from build123d import *

# Parameters (mm, degrees)
BOSS_EXTRUDE1_DEPTH = 24
CUT_EXTRUDE1_DEPTH  = 43
SKETCH7_R           = 12.7
CUT_EXTRUDE4_DEPTH  = 10


with BuildPart() as part:
    # Sketch1 → Boss-Extrude1 (new, symmetric)
    with BuildSketch(Plane.XY):
        with BuildLine():
            Line((0, 41.872855029), (0, -41.872855029))
            ThreePointArc((0, -41.872855029), (5.455474373, -55.600810969), (18.845677428, -61.839515726))
            Line((18.845677428, -61.839515726), (160, -70))
            ThreePointArc((160, -70), (230, 0), (160, 70))
            Line((160, 70), (18.845677428, 61.839515726))
            ThreePointArc((18.845677428, 61.839515726), (5.455474373, 55.600810969), (0, 41.872855029))
        make_face()
    extrude(amount=BOSS_EXTRUDE1_DEPTH, both=True)

    # Sketch2 → Cut-Extrude1 (cut)
    with BuildSketch(Plane(origin=(0, 0, -24), x_dir=(-1, 0, 0), z_dir=(0, 0, -1))):
        with BuildLine():
            Line((-19.134258071, 56.847850552), (-160.141737643, 64.999845465))
            ThreePointArc((-160.141737643, 64.999845465), (-225, 0), (-160.141737643, -64.999845465))
            Line((-160.141737643, -64.999845465), (-19.134258071, -56.847850552))
            ThreePointArc((-19.134258071, -56.847850552), (-9.09160578, -52.168821984), (-5, -41.872855029))
            Line((-5, -41.872855029), (-5, 41.872855029))
            ThreePointArc((-5, 41.872855029), (-9.09160578, 52.168821984), (-19.134258071, 56.847850552))
        make_face()
    extrude(amount=-CUT_EXTRUDE1_DEPTH, mode=Mode.SUBTRACT)

    # Sketch7 → Cut-Extrude4 (cut)
    with BuildSketch(Plane.XY.offset(24)):
        with Locations((50, 0)):
            Circle(SKETCH7_R)
    extrude(amount=-CUT_EXTRUDE4_DEPTH, mode=Mode.SUBTRACT)


solid = part.part
The listing builds one solid part. Answer for the finished solid, in the listing's coordinates (mm). A direction names the side the tool comes from. Coordinates: 2 decimals unless noted, no trailing zeros. Write each loop counter-clockwise with the first axis right and the second up, starting at its lowest first coordinate (ties: lowest second). Pieces come first, ordered by that corner, then holes. Notation, with made-up numbers: M 71.25,22 L 125.25,22 A20 cw 125.25,42 Z; hole C 77.25,25.5 d7. An arc over 180 degrees is marked long. Write each question's results on one line, items separated by ' | '.
Item 1: The part is cut by section B-B on x = 50. Determine the outline of the cut face in (y, z).
Answer below:
outline: M -63.64,-24 L -58.63,-24 L -58.63,19 L -12.7,19 L -12.7,24 L -63.64,24 Z; M 12.7,19 L 58.63,19 L 58.63,-24 L 63.64,-24 L 63.64,24 L 12.7,24 Z
Item 2: The part is cut by section C-C on z = -2.5. Determine the outline of the cut face in (x, y), and give its area (3 significant figures).
Answer below:
outline: M 0,-41.87 A20 ccw 18.85,-61.84 L 160,-70 A70 ccw 160,70 L 18.85,61.84 A20 ccw 0,41.87 Z; hole M 5,-41.87 A15 ccw 19.13,-56.85 L 160.14,-65 A65 ccw 160.14,65 L 19.13,56.85 A15 ccw 5,41.87 Z | area: 3,160 mm2
Item 3: The part is cut by section D-D on y = -46. Determine the outline of the cut face in (x, z), and give its area (3 significant figures).
Answer below:
outline: M 0.43,-24 L 5.58,-24 L 5.58,19 L 205.92,19 L 205.92,-24 L 212.76,-24 L 212.76,24 L 0.43,24 Z | area: 1,580 mm2
Item 4: Which of the six approach directions +Z, -Z, +X, -X, +Y, -Y give full straight-line access (tool end or side, diameter ignored) to faces 1 (the face through (9.2, -52.28, -2.8)), 2 (the face through (88.435, -65.863, 0.336))?
Answer below:
face 1: -Z | face 2: +Z, -Z, -X, -Y
Item 5: For a pull along X with two mould halves and no side action, classify faces 3 (the face through (62.114, 3.815, 21.535)), 4 (the face through (90.411, 65.977, 0.336)), 5 (the face through (113, 1, 24)) as released by +X, released by -X, zero draft, split by the parting line, or undercut.
Answer below:
face 3: undercut | face 4: released by -X | face 5: zero draft
Item 6: Consider probe 1 along Z at (x, y) = (44, 23); probe 2 along X at (y, z) = (13, 16.5); probe 3 along Y at (x, z) = (101, -15.5). Determine where each line is inside the solid, lowest interval first. Write a range as [from, to].
Answer below:
probe 1: [19, 24] | probe 2: [0, 5], [223.69, 228.78] | probe 3: [-66.59, -61.58], [61.58, 66.59]
Item 7: Given P1, Ø8, axis at x = 203, z = -15, coming from the +Y side; P2, Ø2, axis at x = 204.5, z = 7, coming from the -Y side; P3, Ø13, axis at y = -4, z = 3, coming from the +X side; P4, Ø20.5, axis at x = 50, y = 0, coming from the +Z side, each flat-ended and moving along its own axis, determine where each tip first touches the part or whether it passes through.
Answer below:
P1: y = 58.13 | P2: y = -54.84 | P3: x = 230 | P4: through
Item 8: The part is cut by section A-A on y = 0. Determine the outline of the cut face in (x, z), and give its area (3 significant figures).
Answer below:
outline: M 0,-24 L 5,-24 L 5,19 L 37.3,19 L 37.3,24 L 0,24 Z; M 62.7,19 L 225,19 L 225,-24 L 230,-24 L 230,24 L 62.7,24 Z | area: 1,450 mm2
